from build123d import *

# Parameters (mm, degrees)
ESBO_O1_R            = 39
EXTRUS_O1_DEPTH      = 5
EXTRUS_O2_DEPTH      = 50
EXTRUS_O2_DEPTH_BACK = 5
EXTRUS_O11_START     = 5
EXTRUS_O11_DEPTH     = 5
ESBO_O7_R            = 35.5
EXTRUS_O12_DEPTH     = 10
EXTRUS_O13_START     = -3.5
EXTRUS_O13_DEPTH     = 3.5


with BuildPart() as part:
    # Esboço1 → Extrusão1 (new body)
    with BuildSketch(Plane(origin=(0, 0, 0), x_dir=(1, 0, 0), z_dir=(0, 1, 0))):
        with Locations(Location((0, 0, 0), (0, 0, 270))):
            Circle(ESBO_O1_R)
    extrude(amount=EXTRUS_O1_DEPTH)

    # Esboço3 → Extrusão2 (add, two sides: drawn at the far end of the back side and taken through both)
    with BuildSketch(Plane(origin=(0, 5, 0), x_dir=(-1, 0, 0), z_dir=(0, 1, 0)).offset(-EXTRUS_O2_DEPTH_BACK)):
        with BuildLine():
            Line((39, 0), (45, 0))
            ThreePointArc((45, 0), (31.819805153, 31.819805153), (0, 45))
            Line((0, 45), (0, 39))
            ThreePointArc((0, 39), (27.577164466, 27.577164466), (39, 0))
        make_face()
        with BuildLine():
            Line((0, -45), (0, -39))
            ThreePointArc((0, -39), (-27.577164466, -27.577164466), (-39, 0))
            Line((-39, 0), (-45, 0))
            ThreePointArc((-45, 0), (-31.819805153, -31.819805153), (0, -45))
        make_face()
    extrude(amount=EXTRUS_O2_DEPTH + EXTRUS_O2_DEPTH_BACK)

    # Esboço5 → Extrusão11 (add)
    with BuildSketch(Plane.XZ.offset(EXTRUS_O11_START)):
        with BuildLine():
            Line((0, 45), (0, 39))
            ThreePointArc((0, 39), (27.577164466, 27.577164466), (39, 0))
            Line((39, 0), (45, 0))
            ThreePointArc((45, 0), (31.819805153, -31.819805153), (0, -45))
            Line((0, -45), (0, -39))
            ThreePointArc((0, -39), (-27.577164466, -27.577164466), (-39, 0))
            Line((-39, 0), (-45, 0))
            ThreePointArc((-45, 0), (-31.819805153, 31.819805153), (0, 45))
        make_face()
    extrude(amount=-EXTRUS_O11_DEPTH)

    # Esboço7 → Extrusão12 (cut)
    with BuildSketch(Plane(origin=(0, 5, 0), x_dir=(1, 0, 0), z_dir=(0, 1, 0))):
        with Locations(Location((0, 0, 0), (0, 0, 270))):
            Circle(ESBO_O7_R)
    extrude(amount=-EXTRUS_O12_DEPTH, mode=Mode.SUBTRACT)

    # Esboço8 → Extrusão13 (add)
    with BuildSketch(Plane.XZ.offset(5).offset(EXTRUS_O13_START)):
        with BuildLine():
            ThreePointArc((0, 35.5), (-9.188076101, 34.290366833), (-17.75, 30.743901834))
            Line((-17.75, 30.743901834), (-15, 25.980762114))
            ThreePointArc((-15, 25.980762114), (-7.764571353, 28.977774789), (0, 30))
            Line((0, 30), (0, 35.5))
        make_face()
        with BuildLine():
            ThreePointArc((-30.743901834, 17.75), (-34.290366833, 9.188076101), (-35.5, 0))
            Line((-35.5, 0), (-30, 0))
            ThreePointArc((-30, 0), (-28.977774789, 7.764571353), (-25.980762114, 15))
            Line((-25.980762114, 15), (-30.743901834, 17.75))
        make_face()
        with BuildLine():
            Line((0, -30), (0, -35.5))
            ThreePointArc((0, -35.5), (9.188076101, -34.290366833), (17.75, -30.743901834))
            Line((17.75, -30.743901834), (15, -25.980762114))
            ThreePointArc((15, -25.980762114), (7.764571353, -28.977774789), (0, -30))
        make_face()
        with BuildLine():
            Line((25.980762114, -15), (30.743901834, -17.75))
            ThreePointArc((30.743901834, -17.75), (34.290366833, -9.188076101), (35.5, 0))
            Line((35.5, 0), (30, 0))
            ThreePointArc((30, 0), (28.977774789, -7.764571353), (25.980762114, -15))
        make_face()
    extrude(amount=EXTRUS_O13_DEPTH)


solid = part.part
Source: CAD feature listing. Evaluate the final solid. Frame: model axes, mm. A direction names the side the tool comes from. Round coordinates to 2 decimals unless told otherwise and drop trailing zeros. Write each loop counter-clockwise with the first axis right and the second up, starting at its lowest first coordinate (ties: lowest second). Pieces come first, ordered by that corner, then holes. Notation, with made-up numbers: (39, 25) - (93, 25) arc R16 ccw to (93, 49) - close; hole circle Ø10 at (19.5, -37.5). An arc over 180 degrees is marked (long way). Use CSV: the item, a comma, the result in double quotes. Start each with the question number.
(1) Set-up query: faces 1 (the face through (-16.394, -3.226, 28.396)), 2 (the face through (-27.27, 29.65, 27.88)), 3 (the face through (0, 25, -42)), 4 (the face through (0, 25, 42)), 5 (the face through (9, -1.5, -32)). Return all of +Z, -Z, +X, -X, +Y, -Y with unobstructed straight access to the full face (end or side cutting, diameter ignored); none if empty.
(2) Material intervals for probe 1 along Y at (x, z) = (3, 35.5); probe 2 along Z at (x, y) = (-22.5, 3); probe 3 along Z at (x, y) = (-23, 2), sorted ascending. Write a range as [from, to].
(3) Cut plane C-C, the plane x = 28. Return loops of the section in (y, z).
(4) Cut plane D-D, the plane x = -21.5. Return loops of the section in (y, z), and give its area (3 significant figures).
(5) First-contact query: pin 1 Ø10.5 at (x, z) = (11, -28.5) entering from +Y; pin 2 Ø1.8 at (y, z) = (-3.5, -33) entering from -X; pin 3 Ø3 at (y, z) = (33, -42.5) entering from -X. Flat tips, straight axial feed; report the tip coordinate or a pass-through.
(6) Cut plane B-B, the plane z = 4.5. Return loops of the section in (x, y), and give its area (3 significant figures).
(7) Cut plane A-A, the plane y = 26. Return loops of the section in (x, z), and give its area (3 significant figures).
Geometry says:
1,face 1,"+Y, -Y"
1,face 2,"-Z, +X, +Y"
1,face 3,"-Z, -X, +Y, -Y"
1,face 4,"+Z, +X, +Y, -Y"
1,face 5,"+Y"
2,probe 1,"[-5, 5]"
2,probe 2,"[-31.86, -27.46], [27.46, 38.97]"
2,probe 3,"[-31.5, -27.04], [27.04, 38.68]"
3,outline,"(-5, -35.23) - (55, -35.23) - (55, -27.15) - (5, -27.15) - (5, -21.82) - (-5, -21.82) - close; (-5, -16.17) - (-1.5, -16.17) - (-1.5, -10.77) - (-5, -10.77) - close; (-5, 21.82) - (5, 21.82) - (5, 27.15) - (-5, 27.15) - close"
4,outline,"(-5, -32.54) - (5, -32.54) - (5, -28.25) - (-5, -28.25) - close; (-5, 28.25) - (5, 28.25) - (5, 32.54) - (55, 32.54) - (55, 39.53) - (-5, 39.53) - close"
4,area,"505 mm²"
5,pin 1,"y = 5"
5,pin 2,"x = -22.15"
5,pin 3,"x = 0"
6,outline,"(-44.77, -5) - (-29.66, -5) - (-29.66, -1.5) - (-35.21, -1.5) - (-35.21, 5) - (-38.74, 5) - (-38.74, 55) - (-44.77, 55) - close; (35.21, -5) - (38.74, -5) - (38.74, 5) - (35.21, 5) - close"
6,area,"452 mm²"
7,outline,"(-45, 0) - (-39, 0) arc R39 cw to (0, 39) - (0, 45) arc R45 ccw to start; (0, -45) arc R45 ccw to (45, 0) - (39, 0) arc R39 cw to (0, -39) - close"
7,area,"792 mm²"
